For this review, use the dimensioned drawing (mm, ordinates from the lowest corner) and the shaded views. A direction names the side the tool comes from. Round coordinates to 2 decimals unless told otherwise and drop trailing zeros. Write each loop counter-clockwise with the first axis right and the second up, starting at its lowest first coordinate (ties: lowest second). Pieces come first, ordered by that corner, then holes. Notation, with made-up numbers: (70, 18.5) -> (111, 18.5) arc R12 cw to (111, 22.5) -> close; hole circle Ø2 at (-37.5, 78). An arc over 180 degrees is marked (long way). Answer as CSV lines item,"result". Start each with the question number.
Item 1: Wall thickness on probe 1 along Y at (x, z) = (63, 31.5); probe 2 along Z at (x, y) = (14, 37); probe 3 along X at (y, z) = (43, 7): over which ranges is each line inside the solid? List them lowest first. Write a range as from..to.
Item 2: Take a section at A-A on z = 21.15. Give the boundary of the cut face in (x, y), then the cut area to 3 significant figures.
Item 3: Machinability: for the marked faces 5 and 6, which of the approach directions +Z, -Z, +X, -X, +Y, -Y give a long, thin tool a straight path to every point of the face, cutting with its end or side? Answer none if there is none.
Item 4: Mouldability with a two-part tool opening along Y and no side actions: class the marked faces 1, 2, 3 and 4 as +Y half, -Y half, draft (parallel to the pull), parting line (faces both ways), or undercut.
Item 5: Take a section at C-C on y = 35. Give the boundary of the cut face in (x, z), then the cut area to 3 significant figures.
Item 6: Take a section at D-D on x = 14.15. Give the boundary of the cut face in (y, z).
Item 7: Take a section at B-B on x = 76.5. Give the boundary of the cut face in (y, z).
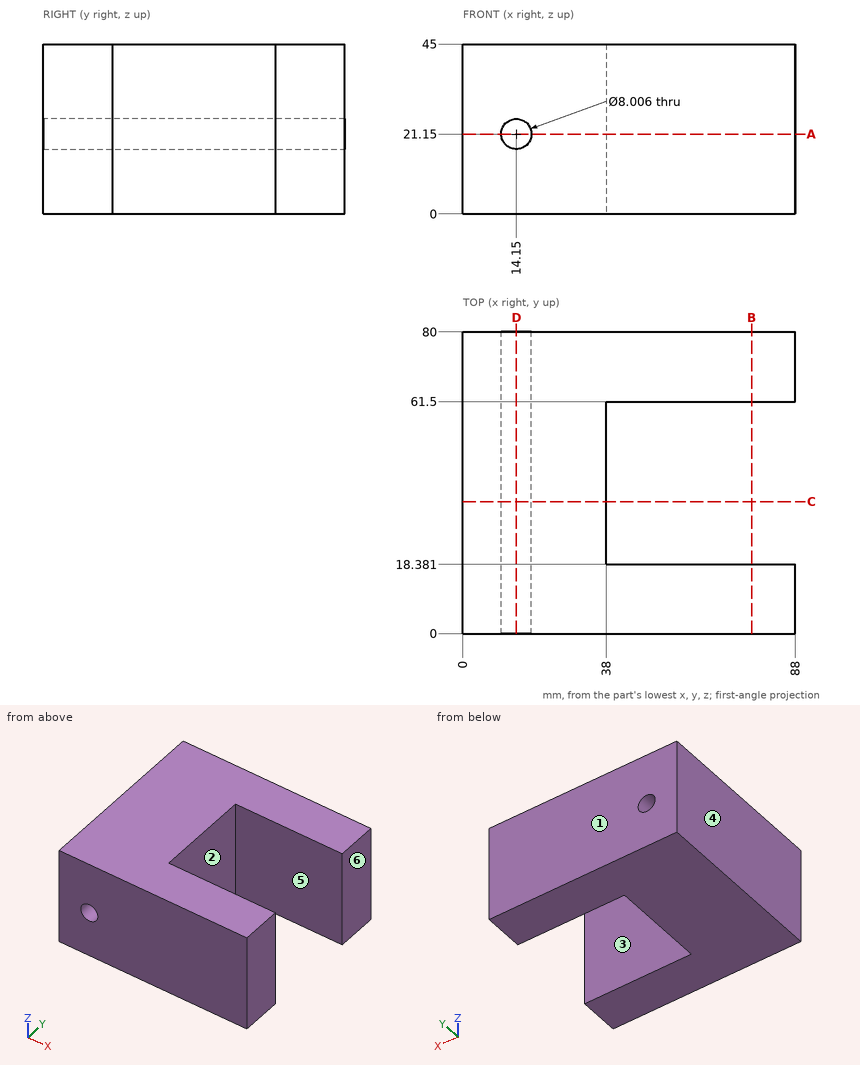
Output values:
1,probe 1,"y = 0..18.38, 61.5..80"
1,probe 2,"z = 0..17.15, 25.15..45"
1,probe 3,"x = 0..38"
2,outline,"(0, 0) -> (10.15, 0) -> (10.15, 80) -> (0, 80) -> close; (18.15, 0) -> (88, 0) -> (88, 18.38) -> (38, 18.38) -> (38, 61.5) -> (88, 61.5) -> (88, 80) -> (18.15, 80) -> close"
2,area,"4,240 mm^2"
3,face 5,"+Z, -Z, +X"
3,face 6,"+Z, -Z, +X, +Y, -Y"
4,face 1,"+Y half"
4,face 2,"undercut"
4,face 3,"undercut"
4,face 4,"draft"
5,outline,"(0, 0) -> (38, 0) -> (38, 45) -> (0, 45) -> close; hole circle Ø8.01 at (14.15, 21.15)"
5,area,"1,660 mm^2"
6,outline,"(0, 0) -> (80, 0) -> (80, 17.15) -> (0, 17.15) -> close; (0, 25.15) -> (80, 25.15) -> (80, 45) -> (0, 45) -> close"
7,outline,"(0, 0) -> (18.38, 0) -> (18.38, 45) -> (0, 45) -> close; (61.5, 0) -> (80, 0) -> (80, 45) -> (61.5, 45) -> close"
